For this review, take the finished solid that the model builds, in its own axes (mm). A direction names the side the tool comes from. Give positions to 0.01 mm unless a question says otherwise; leave off trailing zeros. Order: outer loops, then holes, each group sorted by start corner. A loop starts at its lowest first (then second) coordinate and runs counter-clockwise, first axis right, second up.
from build123d import *

# Parameters (mm, degrees)
SKETCH1_R      = 3.5
BASE_DEPTH     = 3
SKETCH2_R      = 1.6
PEG_DEPTH      = 3
SKETCH5_R      = 4.5
HOLDER_DEPTH   = 3.2
SKETCH8_W      = 12
SKETCH8_H      = 3
CUT_SLOT_DEPTH = 2
FILLET1_R      = 2


with BuildPart() as part:
    # Sketch1 → base (new body)
    with BuildSketch(Plane(origin=(0, 0, 0), x_dir=(1, 0, 0), z_dir=(0, 1, 0))):
        with Locations(Location((0, 0, 0), (0, 0, 270))):
            Circle(SKETCH1_R)
    extrude(amount=BASE_DEPTH)

    # Sketch2 → peg (add)
    with BuildSketch(Plane(origin=(0, 3, 0), x_dir=(1, 0, 0), z_dir=(0, 1, 0))):
        with Locations(Location((0, 0, 0), (0, 0, 270))):
            Circle(SKETCH2_R)
    extrude(amount=PEG_DEPTH)

    # Sketch5 → holder (add)
    with BuildSketch(Plane.XZ):
        with Locations(Location((0, 0, 0), (0, 0, 270))):
            Circle(SKETCH5_R)
    extrude(amount=HOLDER_DEPTH)

    # Sketch6 → Cut-ball (revolve, cut)
    with BuildSketch(Plane(origin=(0, 0, 0), x_dir=(0, 0, -1), z_dir=(1, 0, 0))):
        with BuildLine():
            Line((0, 0.902192429), (0, -5.597807571))
            ThreePointArc((0, -5.597807571), (-3.25, -2.347807571), (0, 0.902192429))
        make_face()
    revolve(axis=Axis((0, 6, 0), (0, -1, 0)), mode=Mode.SUBTRACT)

    # Sketch8 → Cut-slot (cut)
    with BuildSketch(Plane.XZ.offset(3.2)):
        Rectangle(SKETCH8_W, SKETCH8_H)
    extrude(amount=-CUT_SLOT_DEPTH, mode=Mode.SUBTRACT)

    # Fillet1
    # the kernel refuses this fillet: 2 mm, written as the material it takes off along each edge
    with BuildSketch(Plane(origin=(0, -3.2, 0), x_dir=(0, 0, -1), z_dir=(-1, 0, 0))) as fillet1_piece_1:
        with BuildLine():
            CenterArc((2.5, -1.896086641), FILLET1_R, 0, 71.449446556)
            Line((3.136282523, 0), (3.149008174, 0.037921733))
            ThreePointArc((3.149008174, 0.037921733), (3.818141262, 0.04), (4.5, 0.04))
            Line((4.5, 0.04), (4.54, 0))
            Line((4.54, 0), (4.54, -1.896086641))
            Line((4.54, -1.896086641), (4.5, -1.896086641))
        make_face()
    revolve(axis=Axis((0, -3.2, 0), (0, -1, 0)), revolution_arc=130.897979083, mode=Mode.SUBTRACT)
    with BuildSketch(Plane(origin=(0, -3.2, 0), x_dir=(0.7553656278426528, 0, -0.6553035695567931), z_dir=(-0.6553035695567931, 0, -0.7553656278426528))) as fillet1_piece_2:
        with BuildLine():
            CenterArc((2.5, -1.896086641), FILLET1_R, 0, 71.449446556)
            Line((3.136282523, 0), (3.149008174, 0.037921733))
            ThreePointArc((3.149008174, 0.037921733), (3.818141262, 0.04), (4.5, 0.04))
            Line((4.5, 0.04), (4.54, 0))
            Line((4.54, 0), (4.54, -1.896086641))
            Line((4.54, -1.896086641), (4.5, -1.896086641))
        make_face()
    revolve(axis=Axis((0, -3.2, 0), (0, -1, 0)), revolution_arc=261.88534443, mode=Mode.SUBTRACT)
    with BuildSketch(Plane(origin=(0, -3.2, 0), x_dir=(-0.7558765624849457, 0, 0.6547141531125946), z_dir=(0.6547141531125946, 0, 0.7558765624849457))) as fillet1_piece_3:
        with BuildLine():
            CenterArc((2.5, -1.896086641), FILLET1_R, 0, 71.449446556)
            Line((3.136282523, 0), (3.149008174, 0.037921733))
            ThreePointArc((3.149008174, 0.037921733), (3.818141262, 0.04), (4.5, 0.04))
            Line((4.5, 0.04), (4.54, 0))
            Line((4.54, 0), (4.54, -1.896086641))
            Line((4.54, -1.896086641), (4.5, -1.896086641))
        make_face()
    revolve(axis=Axis((0, -3.2, 0), (0, -1, 0)), revolution_arc=130.897979083, mode=Mode.SUBTRACT)


solid = part.part
1) We need section D-D on y = 0.25. Give the boundary of the cut face in (x, z), then the cut area to 3 significant figures.
Answer sheet:
outline: circle Ø7 at (0, 0); hole circle Ø3.91 at (0, 0)
area: 26.5 mm2
2) Draft analysis for pull direction Z (two halves, no side actions). For faces 1 (the face through (-3.5, -2, -1.5)), 2 (the face through (-3.5, -2, 1.5)), 3 (the face through (0, 6, 0)), 4 (the face through (-3.417, 1.479, -0.759)), state which applies: +Z half, -Z half, draft (parallel to the pull), parting line (faces both ways), or undercut.
Answer sheet:
face 1: undercut
face 2: undercut
face 3: draft
face 4: parting line
3) Tool access review of faces 5 (the face through (-1, 3, 2)), 6 (the face through (-4, -1.2, 0)), 7 (the face through (1.352, -0.643, -4.292)): name each direction out of +Z, -Z, +X, -X, +Y, -Y from which nothing blocks a thin tool from reaching the whole face with its end or side.
Answer sheet:
face 5: +Y
face 6: +X, -X, -Y
face 7: +Y, -Y
4) We need section A-A on z = 0. Give the boundary of the cut face in (x, y), then the cut area to 3 significant figures.
Answer sheet:
outline: (-4.5, -1.2) - (-3.04, -1.2) arc R3.25 cw to (3.04, -1.2) - (4.5, -1.2) - (4.5, 0) - (3.5, 0) - (3.5, 3) - (1.6, 3) - (1.6, 6) - (-1.6, 6) - (-1.6, 3) - (-3.5, 3) - (-3.5, 0) - (-4.5, 0) - close
area: 32.1 mm2
5) Clearance check with flat-ended pins moving along their axes: pin 1 (3 mm diameter, centred on y = 2.5, z = -2.5, fed in from +X); pin 2 (2 mm diameter, centred on y = 1.5, z = -3.5, fed in from -X); pin 3 (0.6 mm diameter, centred on x = -3.5, z = 0.5, fed in from -Y). State where each tip first meets the part, or that it passes through.
Answer sheet:
pin 1: stops at x = 3.35
pin 2: stops at x = -2.45
pin 3: stops at y = -1.2
6) To check wall thickness, follow line 1 (X direction, y = 3.5, z = 0); line 2 (X direction, y = -0.5, z = 1.5); line 3 (Z direction, x = -1, y = -0.5). State the ranges of each line that lie inside material, in increasing order.
Answer sheet:
line 1: x = -1.6 to 1.6
line 2: x = -4.24 to -2.21, 2.21 to 4.24
line 3: z = -4.39 to -2.48, 2.48 to 4.39
7) We need section B-B on y = -0.75. Give the boundary of the cut face in (x, z).
Answer sheet:
outline: circle Ø9 at (0, 0); hole circle Ø5.66 at (0, 0)
8) We need section C-C on y = 5.75. Give the boundary of the cut face in (x, z).
Answer sheet:
outline: circle Ø3.2 at (0, 0)
